Part model, mm, in its own coordinate system. A direction names the side the tool comes from. Round coordinates to 2 decimals unless told otherwise and drop trailing zeros. Loops run counter-clockwise (first coordinate to the right, second up) from the corner with the lowest first, then second, coordinate; pieces in that order, holes last. Notation, with made-up numbers: (62, 54) - (90, 54) arc R24 cw to (90, 70) - close; hole circle Ø6 at (26.25, -13). An arc over 180 degrees is marked (long way). Put each result on its own line as item: value.
from build123d import *

# Parameters (mm, degrees)
BOSS_EXTRUDE1_DEPTH = 106


with BuildPart() as part:
    # Sketch1 → Boss-Extrude1 (new body)
    with BuildSketch(Plane.XY):
        with BuildLine():
            Line((-65, 17), (-63.939339828, 15.939339828))
            Line((-63.939339828, 15.939339828), (-62.878679656, 17))
            Line((-62.878679656, 17), (-62.5, 17))
            Line((-62.5, 17), (-61.439339828, 15.939339828))
            Line((-61.439339828, 15.939339828), (-60.378679656, 17))
            Line((-60.378679656, 17), (-60, 17))
            Line((-60, 17), (-58.939339828, 15.939339828))
            Line((-58.939339828, 15.939339828), (-57.878679656, 17))
            Line((-57.878679656, 17), (-57.5, 17))
            Line((-57.5, 17), (-56.439339828, 15.939339828))
            Line((-56.439339828, 15.939339828), (-55.378679656, 17))
            Line((-55.378679656, 17), (-55, 17))
            Line((-55, 17), (-53.939339828, 15.939339828))
            Line((-53.939339828, 15.939339828), (-52.878679656, 17))
            Line((-52.878679656, 17), (-52.5, 17))
            Line((-52.5, 17), (-51.439339828, 15.939339828))
            Line((-51.439339828, 15.939339828), (-50.378679656, 17))
            Line((-50.378679656, 17), (-50, 17))
            Line((-50, 17), (-48.939339828, 15.939339828))
            Line((-48.939339828, 15.939339828), (-47.878679656, 17))
            Line((-47.878679656, 17), (-47.5, 17))
            Line((-47.5, 17), (-46.439339828, 15.939339828))
            Line((-46.439339828, 15.939339828), (-45.378679656, 17))
            Line((-45.378679656, 17), (-45, 17))
            Line((-45, 17), (-43.939339828, 15.939339828))
            Line((-43.939339828, 15.939339828), (-42.878679656, 17))
            Line((-42.878679656, 17), (-42.5, 17))
            Line((-42.5, 17), (-41.439339828, 15.939339828))
            Line((-41.439339828, 15.939339828), (-40.378679656, 17))
            Line((-40.378679656, 17), (-40, 17))
            Line((-40, 17), (-38.939339828, 15.939339828))
            Line((-38.939339828, 15.939339828), (-37.878679656, 17))
            Line((-37.878679656, 17), (-37.5, 17))
            Line((-37.5, 17), (-36.439339828, 15.939339828))
            Line((-36.439339828, 15.939339828), (-35.378679656, 17))
            Line((-35.378679656, 17), (-35, 17))
            Line((-35, 17), (-33.939339828, 15.939339828))
            Line((-33.939339828, 15.939339828), (-32.878679656, 17))
            Line((-32.878679656, 17), (-32.5, 17))
            Line((-32.5, 17), (-31.439339828, 15.939339828))
            Line((-31.439339828, 15.939339828), (-30.378679656, 17))
            Line((-30.378679656, 17), (-30, 17))
            Line((-30, 17), (-28.939339828, 15.939339828))
            Line((-28.939339828, 15.939339828), (-27.878679656, 17))
            Line((-27.878679656, 17), (-27.5, 17))
            Line((-27.5, 17), (-26.439339828, 15.939339828))
            Line((-26.439339828, 15.939339828), (-25.378679656, 17))
            Line((-25.378679656, 17), (-25, 17))
            Line((-25, 17), (-23.939339828, 15.939339828))
            Line((-23.939339828, 15.939339828), (-22.878679656, 17))
            Line((-22.878679656, 17), (-22.5, 17))
            Line((-22.5, 17), (-21.439339828, 15.939339828))
            Line((-21.439339828, 15.939339828), (-20.378679656, 17))
            Line((-20.378679656, 17), (-20, 17))
            Line((-20, 17), (-18.939339828, 15.939339828))
            Line((-18.939339828, 15.939339828), (-17.878679656, 17))
            Line((-17.878679656, 17), (-17.5, 17))
            Line((-17.5, 17), (-16.439339828, 15.939339828))
            Line((-16.439339828, 15.939339828), (-15.378679656, 17))
            Line((-15.378679656, 17), (-15, 17))
            Line((-15, 17), (-13.939339828, 15.939339828))
            Line((-13.939339828, 15.939339828), (-12.878679656, 17))
            Line((-12.878679656, 17), (-12.5, 17))
            Line((-12.5, 17), (-11.439339828, 15.939339828))
            Line((-11.439339828, 15.939339828), (-10.378679656, 17))
            Line((-10.378679656, 17), (-10, 17))
            Line((-10, 17), (-8.939339828, 15.939339828))
            Line((-8.939339828, 15.939339828), (-7.878679656, 17))
            Line((-7.878679656, 17), (-7.5, 17))
            Line((-7.5, 17), (-6.439339828, 15.939339828))
            Line((-6.439339828, 15.939339828), (-5.378679656, 17))
            Line((-5.378679656, 17), (-5, 17))
            Line((-5, 17), (-3.939339828, 15.939339828))
            Line((-3.939339828, 15.939339828), (-2.878679656, 17))
            Line((-2.878679656, 17), (2.5, 17))
            Line((2.5, 17), (3.560660172, 15.939339828))
            Line((3.560660172, 15.939339828), (4.621320344, 17))
            Line((4.621320344, 17), (5, 17))
            Line((5, 17), (6.060660172, 15.939339828))
            Line((6.060660172, 15.939339828), (7.121320344, 17))
            Line((7.121320344, 17), (7.5, 17))
            Line((7.5, 17), (8.560660172, 15.939339828))
            Line((8.560660172, 15.939339828), (9.621320344, 17))
            Line((9.621320344, 17), (10, 17))
            Line((10, 17), (11.060660172, 15.939339828))
            Line((11.060660172, 15.939339828), (12.121320344, 17))
            Line((12.121320344, 17), (12.5, 17))
            Line((12.5, 17), (13.560660172, 15.939339828))
            Line((13.560660172, 15.939339828), (14.621320344, 17))
            Line((14.621320344, 17), (15, 17))
            Line((15, 17), (16.060660172, 15.939339828))
            Line((16.060660172, 15.939339828), (17.121320344, 17))
            Line((17.121320344, 17), (17.5, 17))
            Line((17.5, 17), (18.560660172, 15.939339828))
            Line((18.560660172, 15.939339828), (19.621320344, 17))
            Line((19.621320344, 17), (20, 17))
            Line((20, 17), (21.060660172, 15.939339828))
            Line((21.060660172, 15.939339828), (22.121320344, 17))
            Line((22.121320344, 17), (22.5, 17))
            Line((22.5, 17), (23.560660172, 15.939339828))
            Line((23.560660172, 15.939339828), (24.621320344, 17))
            Line((24.621320344, 17), (25, 17))
            Line((25, 17), (26.060660172, 15.939339828))
            Line((26.060660172, 15.939339828), (27.121320344, 17))
            Line((27.121320344, 17), (27.5, 17))
            Line((27.5, 17), (28.560660172, 15.939339828))
            Line((28.560660172, 15.939339828), (29.621320344, 17))
            Line((29.621320344, 17), (30, 17))
            Line((30, 17), (31.060660172, 15.939339828))
            Line((31.060660172, 15.939339828), (32.121320344, 17))
            Line((32.121320344, 17), (32.5, 17))
            Line((32.5, 17), (33.560660172, 15.939339828))
            Line((33.560660172, 15.939339828), (34.621320344, 17))
            Line((34.621320344, 17), (35, 17))
            Line((35, 17), (36.060660172, 15.939339828))
            Line((36.060660172, 15.939339828), (37.121320344, 17))
            Line((37.121320344, 17), (37.5, 17))
            Line((37.5, 17), (38.560660172, 15.939339828))
            Line((38.560660172, 15.939339828), (39.621320344, 17))
            Line((39.621320344, 17), (40, 17))
            Line((40, 17), (41.060660172, 15.939339828))
            Line((41.060660172, 15.939339828), (42.121320344, 17))
            Line((42.121320344, 17), (42.5, 17))
            Line((42.5, 17), (43.560660172, 15.939339828))
            Line((43.560660172, 15.939339828), (44.621320344, 17))
            Line((44.621320344, 17), (45, 17))
            Line((45, 17), (46.060660172, 15.939339828))
            Line((46.060660172, 15.939339828), (47.121320344, 17))
            Line((47.121320344, 17), (47.5, 17))
            Line((47.5, 17), (48.560660172, 15.939339828))
            Line((48.560660172, 15.939339828), (49.621320344, 17))
            Line((49.621320344, 17), (50, 17))
            Line((50, 17), (51.060660172, 15.939339828))
            Line((51.060660172, 15.939339828), (52.121320344, 17))
            Line((52.121320344, 17), (52.5, 17))
            Line((52.5, 17), (53.560660172, 15.939339828))
            Line((53.560660172, 15.939339828), (54.621320344, 17))
            Line((54.621320344, 17), (55, 17))
            Line((55, 17), (56.060660172, 15.939339828))
            Line((56.060660172, 15.939339828), (57.121320344, 17))
            Line((57.121320344, 17), (57.5, 17))
            Line((57.5, 17), (58.560660172, 15.939339828))
            Line((58.560660172, 15.939339828), (59.621320344, 17))
            Line((59.621320344, 17), (60, 17))
            Line((60, 17), (61.060660172, 15.939339828))
            Line((61.060660172, 15.939339828), (62.121320344, 17))
            Line((62.121320344, 17), (62.5, 17))
            Line((62.5, 17), (63.560660172, 15.939339828))
            Line((63.560660172, 15.939339828), (64.621320344, 17))
            Line((64.621320344, 17), (65, 17))
            ThreePointArc((65, 17), (68.535533906, 15.535533906), (70, 12))
            Line((70, 12), (70, -12))
            ThreePointArc((70, -12), (68.535533906, -15.535533906), (65, -17))
            Line((65, -17), (-65, -17))
            ThreePointArc((-65, -17), (-68.535533906, -15.535533906), (-70, -12))
            Line((-70, -12), (-70, 12))
            ThreePointArc((-70, 12), (-68.535533906, 15.535533906), (-65, 17))
        make_face()
        with BuildLine():
            Line((-64.5, 15.5), (64.5, 15.5))
            ThreePointArc((64.5, 15.5), (67.328427125, 14.328427125), (68.5, 11.5))
            Line((68.5, 11.5), (68.5, -11.5))
            ThreePointArc((68.5, -11.5), (67.328427125, -14.328427125), (64.5, -15.5))
            Line((64.5, -15.5), (-64.5, -15.5))
            ThreePointArc((-64.5, -15.5), (-67.328427125, -14.328427125), (-68.5, -11.5))
            Line((-68.5, -11.5), (-68.5, 11.5))
            ThreePointArc((-68.5, 11.5), (-67.328427125, 14.328427125), (-64.5, 15.5))
        make_face(mode=Mode.SUBTRACT)
    extrude(amount=BOSS_EXTRUDE1_DEPTH)


solid = part.part
1. Pin check, flat tip, straight feed: P1, Ø6, axis at x = 25, y = 10, coming from the +Z side. Stop position of the tip, or through.
A:
P1: passes through
2. Probe line 1 along X through (y, z) = (-9.5, 53.5); line 2 along Y through (x, z) = (-54.5, 42.5); line 3 along X through (y, z) = (-14, 17). List the from-to ranges inside material, lowest first. Write a range as [from, to].
A:
line 1: x = [-70, -68.5], [68.5, 70]
line 2: y = [-17, -15.5], [15.5, 16.5]
line 3: x = [-69.58, -67.62], [67.62, 69.58]
3. Band-saw the part on B-B (x = 0.5). List the corners of the cut face in (y, z).
A:
outline: (-17, 0) - (-15.5, 0) - (-15.5, 106) - (-17, 106) - close; (15.5, 0) - (17, 0) - (17, 106) - (15.5, 106) - close
4. Band-saw the part on A-A (y = 7). List the corners of the cut face in (x, z), plus the area to 3 significant figures.
A:
outline: (-70, 0) - (-68.5, 0) - (-68.5, 106) - (-70, 106) - close; (68.5, 0) - (70, 0) - (70, 106) - (68.5, 106) - close
area: 318 mm²
5. Two-plate mould, pull along X, no slides. Class faces 1 (the flat face through (6, -16, 0)), 2 (the cylindrical face through (67.297, 14.359, 52.258)), 3 (the cylindrical face through (68, 16, 52)): pulls with the +X half, pulls with the -X half, needs draft (parallel to the pull), parting line crosses it, or undercut.
A:
face 1: needs draft
face 2: undercut
face 3: pulls with the +X half
6. Tool access for faces 4 (the flat face through (1, -17, 52)), 5 (the flat face through (1, -15.5, 52)): list every direction of +Z, -Z, +X, -X, +Y, -Y with a clear straight run to the whole face (end or side of a thin tool).
A:
face 4: +Z, -Z, +X, -X, -Y
face 5: +Z, -Z
